Here's how the part is built. I have some questions about the finished solid (model axes, mm). A direction names the side the tool comes from. Coordinates: 2 decimals unless noted, no trailing zeros. Write each loop counter-clockwise with the first axis right and the second up, starting at its lowest first coordinate (ties: lowest second). Pieces come first, ordered by that corner, then holes.
Item 1: If we section it at C-C (z = 1): Count the separate pieces of the cut face and the enclosed holes in it, then the cut area to 3 significant figures.
Item 2: If I drill on line 1 (X direction, y = 0, z = 2.3); line 2 (Y direction, x = -25, z = -5); line 3 (Y direction, x = -1.5, z = -13), over which ranges is the centre line in solid material (lowest first)?
Item 3: I'm going to push flat-ended pins straight in: pin 1 Ø13.5 at (x, y) = (0, 0) entering from -Z; pin 2 Ø2.5 at (x, y) = (-25, -21.5) entering from +Z; pin 3 Ø3 at (x, z) = (22.5, -13) entering from -Y; pin 4 Ø10 at (x, z) = (-11.5, -16) entering from -Y. Where does each tip first touch, or does it pass through?
Item 4: We'd pull the mould along Y, two halves only. Please class faces 1 (the face through (-30, -30.269, -15)), 2 (the face through (-21.746, 17.505, -2.605)), 3 (the face through (8, 11, 5)): +Y half, -Y half, draft (parallel to the pull), parting line (faces both ways), or undercut.
Item 5: For faces 4 (the face through (-24.053, -27.936, -15.28)), 5 (the face through (-11.898, -9.987, 2.465)), 6 (the face through (-25, 20, -10)), 7 (the face through (-3.92, -17.67, -12.98)), which set-ups out of +Z, -Z, +X, -X, +Y, -Y let a thin tool reach every point of the face, with its end or its side?
Item 6: If we section it at A-A (x = -4.5): Please give me the cut outline in (y, z), then the cut area to 3 significant figures.
Item 7: If we section it at D-D (z = -32): Please give me the cut outline in (x, y), then the cut area to 3 significant figures.
Item 8: If we section it at B-B (y = 0): Please give me the cut outline in (x, z), then the cut area to 3 significant figures.
from build123d import *
from build123d.topology import SkipClean

# Parameters (mm, degrees)
SALIENTE_EXTRUIR1_START = -35
SALIENTE_EXTRUIR1_DEPTH = 40
CROQUIS5_R              = 18.1
CORTAR_EXTRUIR1_DEPTH   = 35
CHAFL_N1_SIZE           = 47.117047316
CHAFL_N1_SIZE_2         = 20
TALADRO1_D              = 8.2
TALADRO1_DEPTH          = 15
TALADRO3_D              = 4
MATRIZC2_COUNT          = 4


with BuildPart() as part:
    # Croquis2 → Saliente-Extruir1 (new body)
    with BuildSketch(Plane.XY.offset(SALIENTE_EXTRUIR1_START)):
        with BuildLine():
            Line((0, -11.2), (0, -25.666803753))
            Line((0, -25.666803753), (22.099478046, -25.666803753))
            Line((22.099478046, -25.666803753), (26.062319902, -30.269332556))
            Line((26.062319902, -30.269332556), (33.890912562, -30.269332556))
            Line((33.890912562, -30.269332556), (33.890912562, 26.630335828))
            Line((33.890912562, 26.630335828), (0, 26.630335828))
            Line((0, 26.630335828), (0, 11.2))
            ThreePointArc((0, 11.2), (11.2, 0), (0, -11.2))
        make_face()
    saliente_extruir1 = extrude(amount=SALIENTE_EXTRUIR1_DEPTH)

    # Simetría1: Saliente-Extruir1 across plane
    with SkipClean():  # the faces are left unmerged after this step: merging them gives an invalid solid
        add(saliente_extruir1.mirror(Plane(origin=(0, 0, 0), x_dir=(0, 0, 1), z_dir=(1, 0, 0))))

    # Croquis5 → Cortar-Extruir1 (cut)
    with SkipClean():  # the faces are left unmerged after this step: merging them gives an invalid solid
        with BuildSketch(Plane.XY):
            Circle(CROQUIS5_R)
        extrude(amount=-CORTAR_EXTRUIR1_DEPTH, mode=Mode.SUBTRACT)

    # Chaflán1
    # the kernel refuses this chamfer: 47.117047316, 20 mm, written as the material it takes off along each edge
    with BuildSketch(Plane(origin=(156.034553022, 26.630335828, -35), x_dir=(0, -0.9998864034585262, -0.015072497429863657), z_dir=(-1, 0, 0))) as chafl_n1_piece_1:
        Polygon((CHAFL_N1_SIZE * 0.999886403469, CHAFL_N1_SIZE * 0.01507249743), (-CHAFL_N1_SIZE_2 * 0.0150724974299, CHAFL_N1_SIZE_2 * 0.999886403459), (0, 0), align=None)
    extrude(amount=156.034553022, mode=Mode.SUBTRACT)
    with BuildSketch(Plane(origin=(-156.034553022, 26.630335828, -35), x_dir=(0, -0.9998864034585262, -0.015072497429863657), z_dir=(1, 0, 0))) as chafl_n1_piece_2:
        Polygon((CHAFL_N1_SIZE * 0.999886403469, -CHAFL_N1_SIZE * 0.01507249743), (-CHAFL_N1_SIZE_2 * 0.0150724974299, -CHAFL_N1_SIZE_2 * 0.999886403459), (0, 0), align=None)
    extrude(amount=156.034553022, mode=Mode.SUBTRACT)

    # Taladro1
    with Locations(Plane.XY.offset(5)):
        with Locations((25, -20), (25, 20), (-25, 20), (-25, -20)):
            Hole(TALADRO1_D / 2, depth=TALADRO1_DEPTH)

    # Taladro3 (through all)
    with Locations(Plane.XY.offset(5)):
        with Locations((9.899494937, 9.899494937)):
            taladro3 = Hole(TALADRO3_D / 2)

    # MatrizC2: Taladro3 ×4 about axis
    matrizc2_axis = Axis((0, 0, 0), (0, 0, 1))
    for i in range(1, MATRIZC2_COUNT):
        add(taladro3.rotate(matrizc2_axis, i * 360 / MATRIZC2_COUNT), mode=Mode.SUBTRACT)


solid = part.part
Answer list:
1. separate pieces: 1
1. enclosed holes: 9
1. area: 2,980 mm2
2. line 1: x = -33.89 to -11.2, 11.2 to 33.89
2. line 2: y = -29.04 to -24.1, -15.9 to 15.9, 24.1 to 26.63
2. line 3: y = -25.67 to -18.04, 18.04 to 26.63
3. pin 1: passes through
3. pin 2: stops at z = -10
3. pin 3: stops at y = -27.87
3. pin 4: stops at y = -25.67
4. face 1: -Y half
4. face 2: undercut
4. face 3: draft
5. face 4: +Z, -Z, -Y
5. face 5: +Z, -Z
5. face 6: +Z
5. face 7: -Z
6. outline: (-25.67, -35) - (-20.49, -35) - (-17.53, -33.75) - (-17.53, 0) - (-10.26, 0) - (-10.26, 5) - (-25.67, 5) - close; (10.26, 0) - (17.53, 0) - (17.53, -18.86) - (26.63, -15) - (26.63, 5) - (10.26, 5) - close
6. area: 596 mm2
7. outline: (-33.89, -30.27) - (-26.06, -30.27) - (-22.1, -25.67) - (22.1, -25.67) - (26.06, -30.27) - (33.89, -30.27) - (33.89, -13.42) - (12.15, -13.42) arc R18.1 cw to (-12.15, -13.42) - (-33.89, -13.42) - close
7. area: 842 mm2
8. outline: (-33.89, -26.3) - (-18.1, -26.3) - (-18.1, 0) - (-11.2, 0) - (-11.2, 5) - (-33.89, 5) - close; (11.2, 0) - (18.1, 0) - (18.1, -26.3) - (33.89, -26.3) - (33.89, 5) - (11.2, 5) - close
8. area: 1,060 mm2
